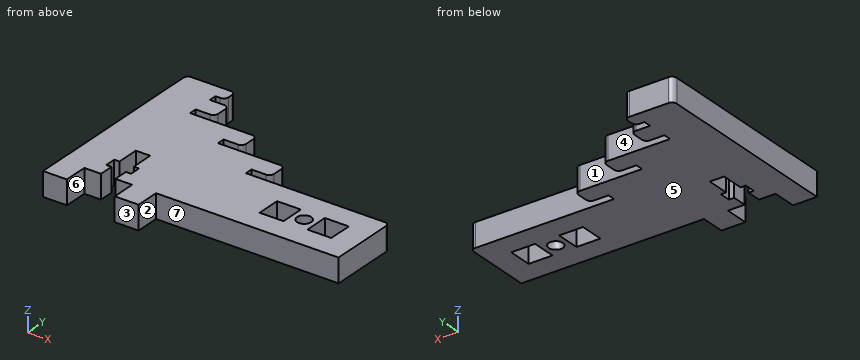
from build123d import *

# Parameters (mm, degrees)
SKETCH1_R           = 1.5
SKETCH1_W           = 5
SKETCH1_H           = 5
BOSS_EXTRUDE1_DEPTH = 5
FILLET3_R           = 1


with BuildPart() as part:
    # Sketch1 → Boss-Extrude1 (new body)
    with BuildSketch(Plane.XY):
        Polygon((0, 5), (0, 19.982808697), (0, 25.3), (0, 30.1), (0, 41.3), (10.2, 41.3), (10.2, 38.3), (8.2, 38.3), (8.2, 36.7), (12.2, 36.7), (12.2, 32.6), (8.2, 32.6), (8.2, 31), (22.2, 31), (22.2, 26.9), (18.2, 26.9), (18.2, 25.3), (32.2, 25.3), (32.2, 21.2), (28.2, 21.2), (28.2, 19.6), (58.2, 19.6), (58.2, 5), (20, 5), (20, 0), (15, 0), (15, 5), (11.5, 5), (11.5, 8), (12.6, 8), (12.6, 10.3), (11.5, 10.3), (11.5, 15), (8.5, 15), (8.5, 10.3), (7.4, 10.3), (7.4, 8), (8.5, 8), (8.5, 5), (5, 5), (5, 0), (0, 0), align=None)
        with Locations((45.7, 12.3)):
            Circle(SKETCH1_R, mode=Mode.SUBTRACT)
        with Locations((40.7, 12.3)):
            Rectangle(SKETCH1_W, SKETCH1_H, mode=Mode.SUBTRACT)
        with Locations((50.7, 12.3)):
            Rectangle(SKETCH1_W, SKETCH1_H, mode=Mode.SUBTRACT)
    extrude(amount=BOSS_EXTRUDE1_DEPTH)

    # Fillet3
    fillet3_edges = [part.edges().sort_by_distance(p)[0] for p in [
        (0, 41.3, 2.5),
        (10.2, 41.3, 2.5),
        (10.2, 38.3, 2.5),
        (12.2, 36.7, 2.5),
        (12.2, 32.6, 2.5),
        (22.2, 31, 2.5),
        (22.2, 26.9, 2.5),
        (32.2, 25.3, 2.5),
        (32.2, 21.2, 2.5),
        (58.2, 19.6, 2.5),
    ]]
    fillet(fillet3_edges, radius=FILLET3_R)


solid = part.part
Read the model definition and answer for the solid it produces. Units are mm, in the model's axes. Face numbers are marked on the shaded views. A direction names the side the tool comes from. Round coordinates to 2 decimals unless told otherwise and drop trailing zeros. Write each loop counter-clockwise with the first axis right and the second up, starting at its lowest first coordinate (ties: lowest second). Pieces come first, ordered by that corner, then holes.
Q1. Straight lines are drawn through the part: line 1 (Y direction, x = 29.5, z = 0.9); line 2 (Y direction, x = 39, z = 2.55); line 3 (X direction, y = 7, z = 0.7). For each, find the intervals that lie inside material, in ascending order.
Values:
line 1: y = 5 to 19.6, 21.2 to 25.3
line 2: y = 5 to 9.8, 14.8 to 19.6
line 3: x = 0 to 8.5, 11.5 to 58.2
Q2. A tool of negligible diameter and unlimited length cuts with its end or side. For the marked faces 5, 6 and 7, from which of +Z, -Z, +X, -X, +Y, -Y can it reach the whole face along a straight path? Write none if from no direction.
Values:
face 5: -Z, +X, -X, +Y, -Y
face 6: +Z, -Z, -Y
face 7: +Z, -Z, +X, -Y
Q3. Find section D-D on z = 3.35. State how many separate pieces and enclosed holes the cut face has, and give its area (3 significant figures).
Values:
separate pieces: 1
enclosed holes: 3
area: 1,210 mm2
Q4. Find section B-B on x = 45.7. Determine the outline of the cut face in (y, z), and give its area (3 significant figures).
Values:
outline: (5, 0) - (10.8, 0) - (10.8, 5) - (5, 5) - close; (13.8, 0) - (19.6, 0) - (19.6, 5) - (13.8, 5) - close
area: 58.0 mm2
Q5. Find section A-A on y = 12.3. Determine the outline of the cut face in (x, z).
Values:
outline: (0, 0) - (8.5, 0) - (8.5, 5) - (0, 5) - close; (11.5, 0) - (38.2, 0) - (38.2, 5) - (11.5, 5) - close; (43.2, 0) - (44.2, 0) - (44.2, 5) - (43.2, 5) - close; (47.2, 0) - (48.2, 0) - (48.2, 5) - (47.2, 5) - close; (53.2, 0) - (58.2, 0) - (58.2, 5) - (53.2, 5) - close
Q6. Find section C-C on y = 7. Determine the outline of the cut face in (x, z).
Values:
outline: (0, 0) - (8.5, 0) - (8.5, 5) - (0, 5) - close; (11.5, 0) - (58.2, 0) - (58.2, 5) - (11.5, 5) - close
Q7. The mould has two halves that part along Y. Classify the marked faces 1, 2, 3 and 4: released by +Y, released by -Y, zero draft, split by the parting line, or undercut.
Values:
face 1: undercut
face 2: zero draft
face 3: released by -Y
face 4: undercut
Q8. Flat-ended cylindrical pins translate along their axes: P1, Ø0.6, axis at y = 23.5, z = 3.5, coming from the +X side; P2, Ø0.8, axis at y = 31.5, z = 2.5, coming from the +X side; P3, Ø2.5, axis at x = 45.7, y = 12.3, coming from the +Z side; P4, Ø2.5, axis at x = 9.5, z = 3.5, coming from the -Y side. Find the tip coordinate at first contact, or state that the pin passes through.
Values:
P1: stops at x = 32.2
P2: stops at x = 8.2
P3: passes through
P4: stops at y = 5
